Job drawing, mm, ordinate dimensions from the low corner. One solid piece. Coordinates: 2 decimals unless noted, no trailing zeros. Order: outer loops, then holes, each group sorted by start corner. A loop starts at its lowest first (then second) coordinate and runs counter-clockwise, first axis right, second up. Notation, with made-up numbers: (44.25, -18) - (63.25, -18) arc R20 ccw to (63.25, 13) - close; hole circle Ø11 at (8.25, 64.25). An arc over 180 degrees is marked (long way). Use a Markdown table: item, result. Add a question column.
1) Saw through at B-B on x = 131. List the corners of the cut face in (y, z) (1 decimal), then the cut area to 3 significant figures.
2) Wall check: L1, parallel to Y at x = 123.5, z = 95 (1 decimal); L2, parallel to Z at x = 79, y = 10 (1 decimal); L3, parallel to X at y = 4, z = 70.5 (1 decimal). Give the ranges that are in metal, low to high. Write a range as [from, to].
3) Saw through at A-A on z = 73. Count the separate pieces of the cut face and the enclosed holes in it.
4) Two-plate mould, pull along Z, no slides. Class the marked faces 1 and 2: +Z half, -Z half, draft (parallel to the pull), parting line (faces both ways), or undercut.
5) Saw through at D-D on z = 40.5. List the corners of the cut face in (x, y) (1 decimal).
6) Drop flat-ended pins along their axis: P1, Ø10, axis at x = 104.5, z = 67.5, coming from the -Y side (1 decimal); P2, Ø12, axis at x = 28, z = 59.5, coming from the +Y side; P3, Ø3, axis at x = 76.5, y = 7.5, coming from the -Z side; P4, Ø7.5, axis at x = 11.91, z = 75.41, coming from the +Y side. Give the stop position or say it passes through.
7) Saw through at C-C on y = 5.75. List the corners of the cut face in (x, z) (1 decimal).
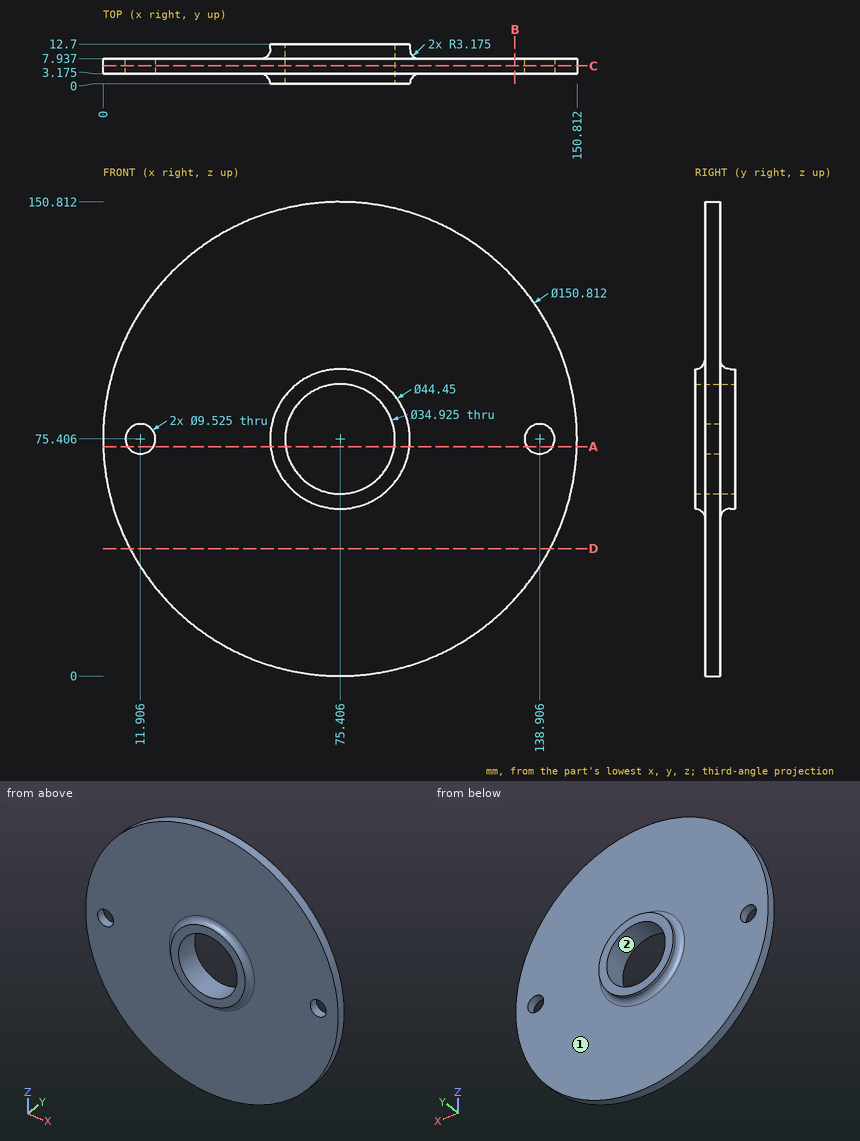
Results are:
| question | item | result |
|---|---|---|
| 1 | outline | (3.2, 24.5) - (7.9, 24.5) - (7.9, 126.4) - (3.2, 126.4) - close |
| 1 | area | 485 mm2 |
| 2 | L1 | [3.2, 7.9] |
| 2 | L2 | [53.3, 58.3], [92.5, 97.5] |
| 2 | L3 | [0.2, 58.6], [92.2, 150.7] |
| 3 | separate pieces | 4 |
| 3 | enclosed holes | 0 |
| 4 | face 1 | draft |
| 4 | face 2 | undercut |
| 5 | outline | (8.6, 3.2) - (142.2, 3.2) - (142.2, 7.9) - (8.6, 7.9) - close |
| 6 | P1 | y = 3.2 |
| 6 | P2 | y = 7.94 |
| 6 | P3 | z = 0 |
| 6 | P4 | through |
| 7 | outline | circle Ø150.8 at (75.4, 75.4); hole circle Ø9.5 at (11.9, 75.4); hole circle Ø34.9 at (75.4, 75.4); hole circle Ø9.5 at (138.9, 75.4) |
